Geometry check sheet. Reference: the model listing, model coordinates, mm. Face numbers are marked on the shaded views. A direction names the side the tool comes from. Give positions to 0.01 mm unless a question says otherwise; leave off trailing zeros. Write each loop counter-clockwise with the first axis right and the second up, starting at its lowest first coordinate (ties: lowest second). Pieces come first, ordered by that corner, then holes. Notation, with made-up numbers: M -39.5,-22.5 L 4.5,-22.5 A16 cw 4.5,-13.5 Z; hole C 52.25,-36 d1. An arc over 180 degrees is marked long. Write each question's results on one line, items separated by ' | '.
```python
from build123d import *

# Parameters (mm, degrees)
SKETCH1_R            = 28.1
BOSS_EXTRUDE2_DEPTH  = 24
CUT_EXTRUDE2_DEPTH   = 21.5
SKETCH4_R            = 3
CUT_EXTRUDE3_DEPTH   = 9.5
SKETCH6_R            = 6.025
CUT_EXTRUDE4_DEPTH   = 6.2
SKETCH7_W            = 56.2
SKETCH7_H            = 56.2
BOSS_EXTRUDE3_DEPTH  = 56.2
SKETCH8_W            = 56.2
SKETCH8_H            = 56.2
BOSS_EXTRUDE4_DEPTH  = 14.14
SKETCH10_W           = 56.2
SKETCH10_H           = 56.2
BOSS_EXTRUDE5_DEPTH  = 10
SKETCH11_W           = 10
SKETCH11_H           = 56.2
BOSS_EXTRUDE6_DEPTH  = 146.9
SKETCH12_W           = 10
SKETCH12_H           = 56.2
BOSS_EXTRUDE7_DEPTH  = 126.9
SKETCH13_W           = 10
SKETCH13_H           = 56.2
BOSS_EXTRUDE8_DEPTH  = 146.9
SKETCH14_W           = 10
SKETCH14_H           = 56.2
BOSS_EXTRUDE9_DEPTH  = 126.9
SKETCH15_W           = 10
SKETCH15_H           = 56.2
BOSS_EXTRUDE10_DEPTH = 25
SKETCH16_W           = 10
SKETCH16_H           = 56.2
BOSS_EXTRUDE11_DEPTH = 25
SKETCH17_W           = 56.2
SKETCH17_H           = 10
BOSS_EXTRUDE12_DEPTH = 25
SKETCH18_W           = 56.2
SKETCH18_H           = 10
BOSS_EXTRUDE13_DEPTH = 25
SKETCH19_W           = 51.2
SKETCH19_H           = 51.2
CUT_EXTRUDE5_DEPTH   = 63.7
SKETCH23_W           = 330
SKETCH23_H           = 16.2
CUT_EXTRUDE7_DEPTH   = 5
SKETCH24_W           = 16.2
SKETCH24_H           = 290
CUT_EXTRUDE8_DEPTH   = 5
SKETCH25_W           = 16.2
SKETCH25_H           = 16.2
CUT_EXTRUDE12_DEPTH  = 25


with BuildPart() as part:
    # Sketch1 → Boss-Extrude2 (new body)
    with BuildSketch(Plane.XY):
        Circle(SKETCH1_R)
    extrude(amount=BOSS_EXTRUDE2_DEPTH)

    # Sketch3 → Cut-Extrude2 (cut)
    with BuildSketch(Plane(origin=(0, 0, 0), x_dir=(-1, 0, 0), z_dir=(0, 0, -1))):
        with BuildLine():
            Line((-1.661801922, 2.5), (1.661801922, 2.5))
            ThreePointArc((1.661801922, 2.5), (0, -3.001930317), (-1.661801922, 2.5))
        make_face()
    extrude(amount=-CUT_EXTRUDE2_DEPTH, mode=Mode.SUBTRACT)

    # Sketch4 → Cut-Extrude3 (cut)
    with BuildSketch(Plane(origin=(0, 0, 0), x_dir=(-1, 0, 0), z_dir=(0, 0, -1))):
        Circle(SKETCH4_R)
    extrude(amount=-CUT_EXTRUDE3_DEPTH, mode=Mode.SUBTRACT)

    # Sketch6 → Cut-Extrude4 (cut)
    with BuildSketch(Plane(origin=(0, 0, 0), x_dir=(-1, 0, 0), z_dir=(0, 0, -1))):
        Circle(SKETCH6_R)
    extrude(amount=-CUT_EXTRUDE4_DEPTH, mode=Mode.SUBTRACT)

    # Sketch7 → Boss-Extrude3 (add)
    with BuildSketch(Plane.XY.offset(24)):
        Rectangle(SKETCH7_W, SKETCH7_H)
    extrude(amount=BOSS_EXTRUDE3_DEPTH)

    # Sketch8 → Boss-Extrude4 (add)
    with BuildSketch(Plane(origin=(28.1, 0, 0), x_dir=(0, 0, -1), z_dir=(1, 0, 0))):
        with Locations((-52.1, 0)):
            Rectangle(SKETCH8_W, SKETCH8_H)
    extrude(amount=BOSS_EXTRUDE4_DEPTH)

    # Sketch10 → Boss-Extrude5 (add)
    with BuildSketch(Plane(origin=(42.24, 0, 0), x_dir=(0, 0, -1), z_dir=(1, 0, 0))):
        with Locations((-52.1, 0)):
            Rectangle(SKETCH10_W, SKETCH10_H)
    extrude(amount=BOSS_EXTRUDE5_DEPTH)

    # Sketch11 → Boss-Extrude6 (add)
    with BuildSketch(Plane.XY.offset(80.2)):
        with Locations((47.24, 0)):
            Rectangle(SKETCH11_W, SKETCH11_H)
    extrude(amount=BOSS_EXTRUDE6_DEPTH)

    # Sketch12 → Boss-Extrude7 (add)
    with BuildSketch(Plane(origin=(0, 28.1, 0), x_dir=(1, 0, 0), z_dir=(0, 1, 0))):
        with Locations((47.24, -52.1)):
            Rectangle(SKETCH12_W, SKETCH12_H)
    extrude(amount=BOSS_EXTRUDE7_DEPTH)

    # Sketch13 → Boss-Extrude8 (add)
    with BuildSketch(Plane(origin=(0, 0, 24), x_dir=(-1, 0, 0), z_dir=(0, 0, -1))):
        with Locations((-47.24, 0)):
            Rectangle(SKETCH13_W, SKETCH13_H)
    extrude(amount=BOSS_EXTRUDE8_DEPTH)

    # Sketch14 → Boss-Extrude9 (add)
    with BuildSketch(Plane(origin=(0, -28.1, 0), x_dir=(-1, 0, 0), z_dir=(0, -1, 0))):
        with Locations((-47.24, -52.1)):
            Rectangle(SKETCH14_W, SKETCH14_H)
    extrude(amount=BOSS_EXTRUDE9_DEPTH)

    # Sketch15 → Boss-Extrude10 (add)
    with BuildSketch(Plane(origin=(52.24, 0, 0), x_dir=(0, 0, -1), z_dir=(1, 0, 0))):
        with Locations((-222.1, 0)):
            Rectangle(SKETCH15_W, SKETCH15_H)
    extrude(amount=BOSS_EXTRUDE10_DEPTH)

    # Sketch16 → Boss-Extrude11 (add)
    with BuildSketch(Plane(origin=(52.24, 0, 0), x_dir=(0, 0, -1), z_dir=(1, 0, 0))):
        with Locations((117.9, 0)):
            Rectangle(SKETCH16_W, SKETCH16_H)
    extrude(amount=BOSS_EXTRUDE11_DEPTH)

    # Sketch17 → Boss-Extrude12 (add)
    with BuildSketch(Plane(origin=(52.24, 0, 0), x_dir=(0, 0, -1), z_dir=(1, 0, 0))):
        with Locations((-52.1, 150)):
            Rectangle(SKETCH17_W, SKETCH17_H)
    extrude(amount=BOSS_EXTRUDE12_DEPTH)

    # Sketch18 → Boss-Extrude13 (add)
    with BuildSketch(Plane(origin=(52.24, 0, 0), x_dir=(0, 0, -1), z_dir=(1, 0, 0))):
        with Locations((-52.1, -150)):
            Rectangle(SKETCH18_W, SKETCH18_H)
    extrude(amount=BOSS_EXTRUDE13_DEPTH)

    # Sketch19 → Cut-Extrude5 (cut)
    with BuildSketch(Plane.ZY.offset(28.1)):
        with Locations((52.1, 0)):
            Rectangle(SKETCH19_W, SKETCH19_H)
    extrude(amount=-CUT_EXTRUDE5_DEPTH, mode=Mode.SUBTRACT)

    # Cut-Sweep2: sweep along a path in Sketch20
    with BuildLine(Plane(origin=(0, 0, 0), x_dir=(-1, 0, 0), z_dir=(0, 0, -1))) as cut_sweep2_path:
        ThreePointArc((0, 15), (-10.606601718, 10.606601718), (-15, 0))
    # 3DSketch2 → Cut-Sweep2 (sweep, cut)
    with BuildSketch(Plane(origin=(0, 15, 0), x_dir=(0, 0.17521220324553322, 0.9845306921746249), z_dir=(-1, 0, 0))):
        Polygon((0, 0), (1.314091524, 7.383980191), (42.805237655, 0), (41.491146131, -7.383980191), align=None)
    sweep(path=cut_sweep2_path.line, mode=Mode.SUBTRACT)

    # Sketch23 → Cut-Extrude7 (cut)
    with BuildSketch(Plane(origin=(52.24, 0, 0), x_dir=(0, 0, -1), z_dir=(1, 0, 0))):
        with Locations((-52.1, 0)):
            Rectangle(SKETCH23_W, SKETCH23_H)
    extrude(amount=-CUT_EXTRUDE7_DEPTH, mode=Mode.SUBTRACT)

    # Sketch24 → Cut-Extrude8 (cut)
    with BuildSketch(Plane(origin=(52.24, 0, 0), x_dir=(0, 0, -1), z_dir=(1, 0, 0))):
        with Locations((-52.1, 0)):
            Rectangle(SKETCH24_W, SKETCH24_H)
    extrude(amount=-CUT_EXTRUDE8_DEPTH, mode=Mode.SUBTRACT)

    # Sketch25 → Cut-Extrude12 (cut)
    with BuildSketch(Plane(origin=(47.24, 0, 0), x_dir=(0, 0, -1), z_dir=(1, 0, 0))):
        with Locations((-52.1, 0)):
            Rectangle(SKETCH25_W, SKETCH25_H)
    extrude(amount=-CUT_EXTRUDE12_DEPTH, mode=Mode.SUBTRACT)


solid = part.part
```
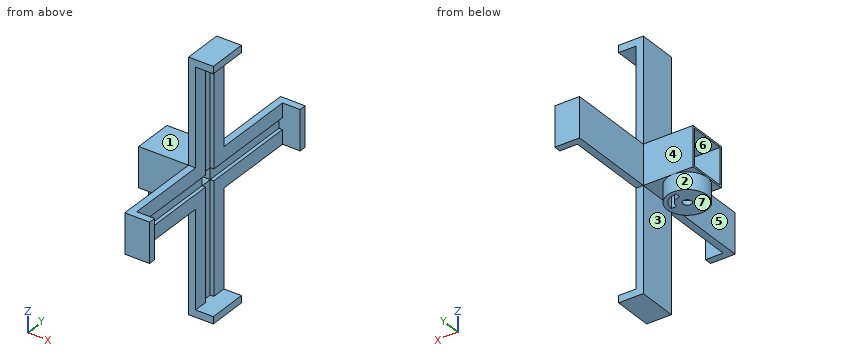
Q1. Access from +Z, -Z, +X, -X, +Y, -Y to the whole of each face (thin tool, end or side, straight path). Record for the marked faces 1, 2, 3 and 4.
Answer key:
face 1: +Z, -X, +Y, -Y | face 2: -Z | face 3: -Z, +Y, -Y | face 4: +Z, -Z, -X, +Y
Q2. Section check A-A (x = 70). Enter the section's corners in (y, z).
Answer key:
outline: M -155,24 L -145,24 L -145,80.2 L -155,80.2 Z; M -28.1,-122.9 L 28.1,-122.9 L 28.1,-112.9 L -28.1,-112.9 Z; M -28.1,217.1 L 28.1,217.1 L 28.1,227.1 L -28.1,227.1 Z; M 145,24 L 155,24 L 155,80.2 L 145,80.2 Z
Q3. Depth check by flat-ended pin: P1, Ø6, axis at x = 55, z = -29.5, coming from the -Y side; P2, Ø8, axis at y = -74, z = 48.5, coming from the +X side; P3, Ø8, axis at x = 0, y = 0, coming from the -Z side. Enter the tip coordinate at first touch or a pass-through.
Answer key:
P1: stops at y = -28.1 | P2: stops at x = 47.24 | P3: stops at z = 6.2
Q4. Section check C-C (z = 142). Enter the section's corners in (x, y).
Answer key:
outline: M 42.24,-28.1 L 52.24,-28.1 L 52.24,-8.1 L 47.24,-8.1 L 47.24,8.1 L 52.24,8.1 L 52.24,28.1 L 42.24,28.1 Z
Q5. Release check for a two-part mould opening along Z. For the marked faces 5, 6 and 7 record: released by +Z, released by -Z, zero draft, split by the parting line, or undercut.
Answer key:
face 5: zero draft | face 6: undercut | face 7: released by -Z
Q6. Section check B-B (y = 102). Enter the section's corners in (x, z).
Answer key:
outline: M 42.24,24 L 52.24,24 L 52.24,44 L 47.24,44 L 47.24,60.2 L 52.24,60.2 L 52.24,80.2 L 42.24,80.2 Z
Q7. Material ranges on probe 1 along Z at (x, y) = (-6.5, 14); probe 2 along Y at (x, z) = (-8.5, 75); probe 3 along Z at (x, y) = (48, 91), recorded low to high. Write a range as [from, to].
Answer key:
probe 1: z = [0, 26.5], [77.7, 80.2] | probe 2: y = [-28.1, -25.6], [25.6, 28.1] | probe 3: z = [24, 44], [60.2, 80.2]
